Geometry check sheet. Reference: drawing and pictorial views, mm from the part's lowest x, y, z. Give positions to 0.01 mm unless a question says otherwise; leave off trailing zeros. Loops run counter-clockwise (first coordinate to the right, second up) from the corner with the lowest first, then second, coordinate; pieces in that order, holes last. Notation, with made-up numbers: (48.25, 52.5) -> (103.25, 52.5) arc R8 ccw to (103.25, 62.5) -> close; hole circle Ø9 at (14.25, 67). An arc over 180 degrees is marked (long way). One line per item, written item: value. Start each with the question number.
(1) Sectioned sample at A-A, the plane y = 12. Record the cut outline in (x, z), then the cut area to 3 significant figures.
(2) Sectioned sample at D-D, the plane z = 43. Record the cut outline in (x, y), then the cut area to 3 significant figures.
(3) Draft check along Z on the marked faces 1, 2, 3 and 4. Enter one of: pulls with the +Z half, pulls with the -Z half, needs draft (parallel to the pull), parting line crosses it, or undercut.
(4) Sectioned sample at C-C, the plane x = 7. Record the cut outline in (y, z).
(5) Scan lines: line 1 along Z through (x, y) = (4.5, 31); line 2 along Y through (x, z) = (7.5, 89); line 3 along Y through (x, z) = (4.75, 45). Record each from-to range of solid material in increasing order. Write a range as from..to.
(6) Sectioned sample at B-B, the plane z = 89. Record the cut outline in (x, y).
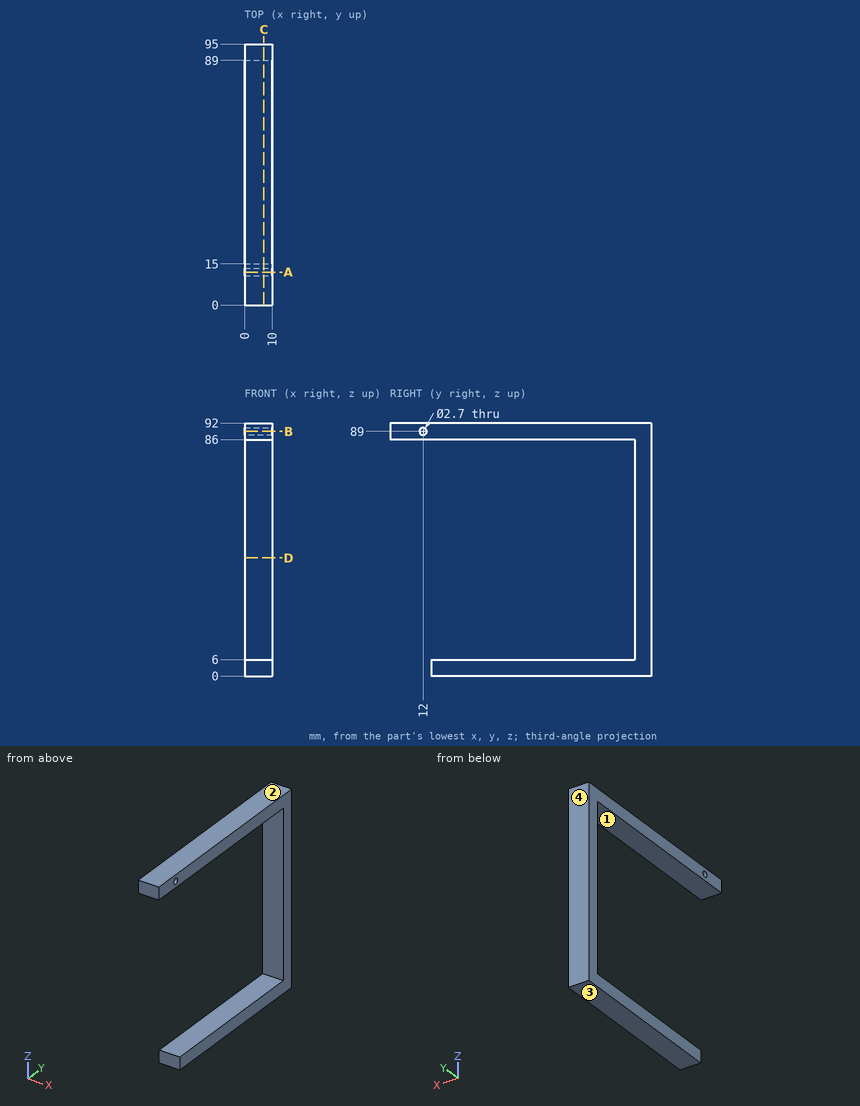
Calculated:
1. outline: (0, 86) -> (10, 86) -> (10, 87.65) -> (0, 87.65) -> close; (0, 90.35) -> (10, 90.35) -> (10, 92) -> (0, 92) -> close
1. area: 33.0 mm2
2. outline: (0, 89) -> (10, 89) -> (10, 95) -> (0, 95) -> close
2. area: 60.0 mm2
3. face 1: undercut
3. face 2: pulls with the +Z half
3. face 3: pulls with the -Z half
3. face 4: needs draft
4. outline: (0, 86) -> (89, 86) -> (89, 6) -> (15, 6) -> (15, 0) -> (95, 0) -> (95, 92) -> (0, 92) -> close; hole circle Ø2.7 at (12, 89)
5. line 1: z = 0..6, 86..92
5. line 2: y = 0..10.65, 13.35..95
5. line 3: y = 89..95
6. outline: (0, 0) -> (10, 0) -> (10, 10.65) -> (0, 10.65) -> close; (0, 13.35) -> (10, 13.35) -> (10, 95) -> (0, 95) -> close
